Autodesk Fusion 360 part; units mm, degrees
sketch "Sketch1" plane through (0, 0, 0) normal (0, 1, 0) x (1, 0, 0)
  line L0 (0, 0) -> (6, 0)
  line L1 (6, 0) -> (6, -150)
  line L2 (6, -150) -> (0, -150)
  line L3 (0, -150) -> (0, 0)
  line L4 (0, -150) -> (6, -139.6077)
  dimension "d1" = 12
  dimension "d2" = 150
  dimension "d3" = 30
revolve "Revolve1" add sketch "Sketch1" angle 360 about axis through (0, 0, 150) along (0, 0, -1) contours L0 L1 L3 L4
hole "Hole1" at (0, 0, 0) direction (0, 0, 1) diameter 5.035 depth 15 tip angle 118
chamfer "Chamfer1" distance 0.5 angle 45 1 edges at (-5.594, -2.1697, 0)
Build history of the part. All positions in model axes, mm. Give positions to 0.01 mm unless a question says otherwise; leave off trailing zeros. Loops run counter-clockwise (first coordinate to the right, second up) from the corner with the lowest first, then second, coordinate; pieces in that order, holes last. Notation, with made-up numbers: (10.5, 88.25) - (22.5, 88.25) arc R31 cw to (22.5, 118.25) - close; hole circle Ø7 at (64, 24.25). An arc over 180 degrees is marked (long way). Write item = value, one per line. Start each with the question number.
1) Probe probe 1 along X at (y, z) = (0, 3.75); probe 2 along Y at (x, z) = (0.5, 46). List the from-to ranges inside material, lowest first. Write a range as from..to.
2) Band-saw the part on A-A on z = 25.5. Give the cut face in (x, y), plus the area to 3 significant figures.
3) Drop flat-ended pins along their axis: pin 1 Ø4 at (x, y) = (0, 0) entering from -Z; pin 2 Ø1 at (x, y) = (3, 0) entering from -Z; pin 3 Ø4 at (x, y) = (-2.5, 1.5) entering from +Z. Give the stop position or say it passes through.
4) Pull direction Y, two halves, no side cores. Call faces 1 (the flat face through (-3, 0, 0)), 2 (the conical face through (2.266, -0.713, 145.886)), 3 (the conical face through (-0.43, -0.09, 16.25)), 4 (the cylindrical face through (-2.5, -0.3, 7.6)): +Y half, -Y half, draft (parallel to the pull), parting line (faces both ways), or undercut.
Final values:
q1.probe_1 = -6..-2.52, 2.52..6
q1.probe_2 = -5.98..5.98
q2.outline = circle Ø12 at (0, 0)
q2.area = 113 mm²
q3.pin_1 = 15.31
q3.pin_2 = 0
q3.pin_3 = 148.41
q4.face_1 = draft
q4.face_2 = parting line
q4.face_3 = undercut
q4.face_4 = undercut
